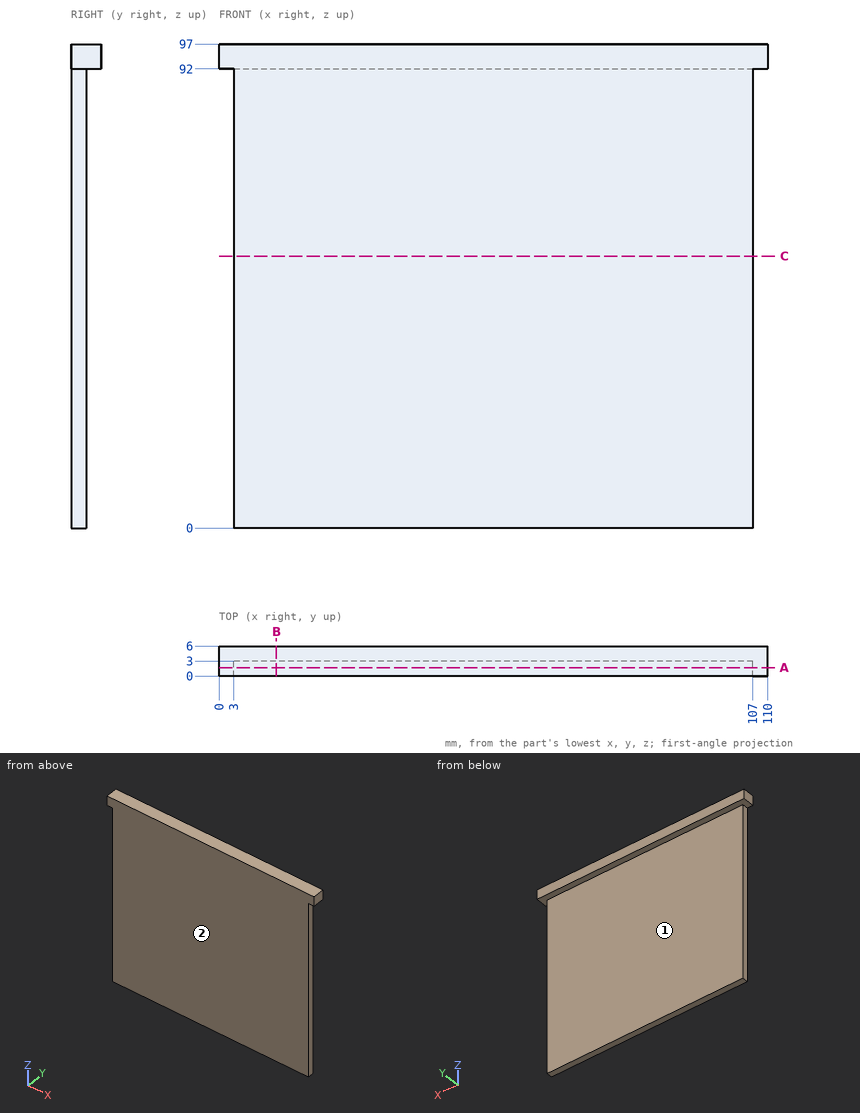
Can you work these out from the drawing? Everything is in mm from the part's minimum corner. A direction names the side the tool comes from. Coordinates: 2 decimals unless noted, no trailing zeros. Write each loop counter-clockwise with the first axis right and the second up, starting at its lowest first coordinate (ties: lowest second). Pieces come first, ordered by that corner, then holes. Notation, with made-up numbers: (1.5, 60) -> (41.5, 60) arc R23 cw to (41.5, 75) -> close; hole circle Ø8 at (-23.5, 84). An arc over 180 degrees is marked (long way). Write each question's results on one line, items separated by ' | '. Start each with the question number.
Item 1: If we section it at A-A, the plane y = 1.7: Write out the boundary of the cut face in (x, z).
Item 2: If we section it at C-C, the plane z = 54.5: Write out the boundary of the cut face in (x, y), and give its area (3 significant figures).
Item 3: I'm going to push flat-ended pins straight in: P1, Ø3, axis at y = 3, z = 78.5, coming from the +X side; P2, Ø5, axis at x = 37.5, z = 20, coming from the +Y side; P3, Ø0.9, axis at y = 1.5, z = 56.5, coming from the -X side. Where does each tip first touch, or does it pass through?
Item 4: Please list where these lines run through material, in increasing order: probe 1 along Y at (x, z) = (31, 35.5); probe 2 along Z at (x, y) = (88, 5.3); probe 3 along X at (y, z) = (2.55, 23).
Item 5: If we section it at B-B, the plane x = 11.5: Write out the boundary of the cut face in (y, z), and give its area (3 significant figures).
Item 6: On a 3-axis mill with a long thin cutter (end or side, diameter ignored), from which of +Z, -Z, +X, -X, +Y, -Y can I reach the whole of each face in a straight line? I mean the marked faces 1 and 2. Say none if no direction works.
Answer block:
1) outline: (0, 92) -> (3, 92) -> (3, 0) -> (107, 0) -> (107, 92) -> (110, 92) -> (110, 97) -> (0, 97) -> close
2) outline: (3, 0) -> (107, 0) -> (107, 3) -> (3, 3) -> close | area: 312 mm²
3) P1: x = 107 | P2: y = 3 | P3: x = 3
4) probe 1: 0 to 3 | probe 2: 92 to 97 | probe 3: 3 to 107
5) outline: (0, 0) -> (3, 0) -> (3, 92) -> (6, 92) -> (6, 97) -> (0, 97) -> close | area: 306 mm²
6) face 1: -Z, +X, -X, +Y | face 2: +Z, -Z, +X, -X, -Y
